Check sheet for the drawn part. Datum: minimum x, y, z corner. Units: mm. A direction names the side the tool comes from. Coordinates: 2 decimals unless noted, no trailing zeros. Write each loop counter-clockwise with the first axis right and the second up, starting at its lowest first coordinate (ties: lowest second). Pieces come first, ordered by that corner, then holes. Notation, with made-up numbers: (-20.75, 71.5) - (-1.75, 71.5) arc R21 cw to (-1.75, 79.5) - close; hole circle Ø11 at (-37.75, 39.25). An arc over 180 degrees is marked (long way). Use CSV: the item, a comma, the result in double quotes. Start each with the question number.
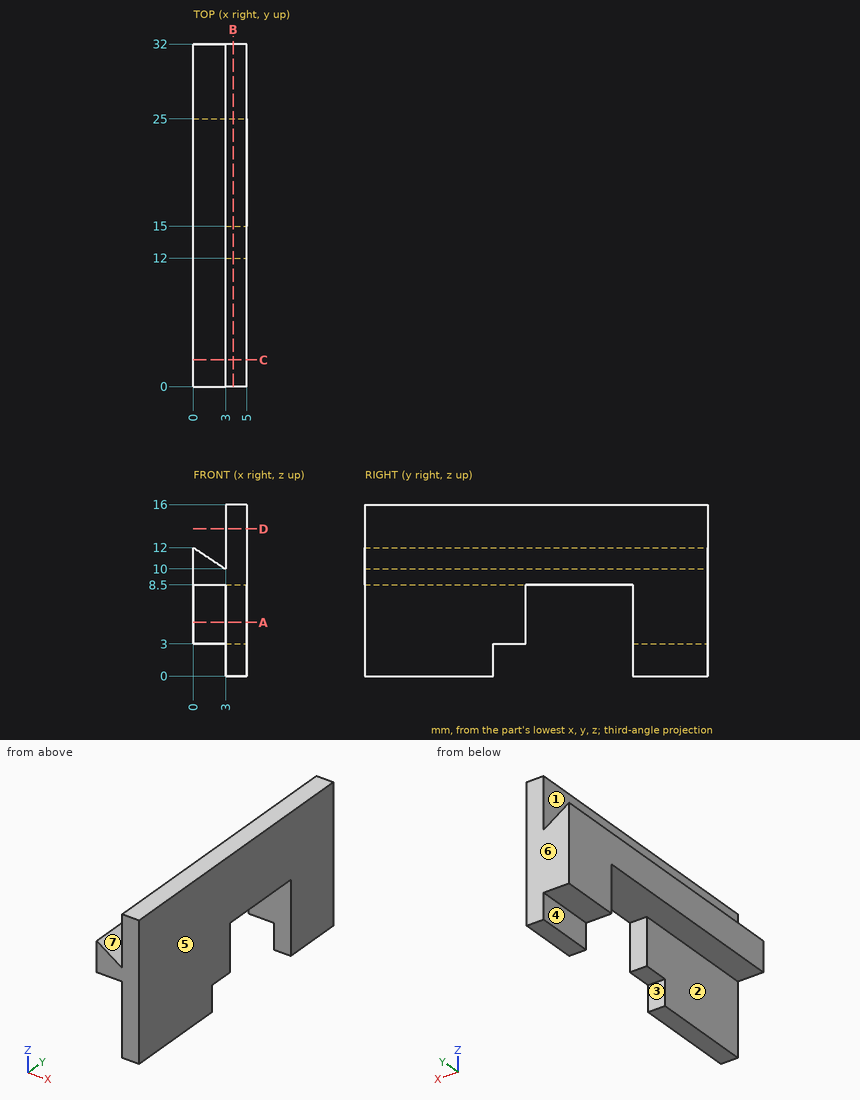
Q1. Cross-section at D-D (z = 13.75). Record the cut outline in (x, y), plus the area to 3 significant figures.
Q2. Cross-section at C-C (y = 2.5). Record the cut outline in (x, z), plus the area to 3 significant figures.
Q3. Tool access check on the marked faces 1, 2, 3 and 4. Record the directions out of +Z, -Z, +X, -X, +Y, -Y that give a thin tool (end or side, any length) a straight path to the whole face; none if there is none.
Q4. Cross-section at A-A (z = 5). Record the cut outline in (x, y).
Q5. Gauge pin test, flat ends, axial feed: pin 1 (2 mm diameter, centred on x = 4.5, y = 13.5, fed in from -Z); pin 2 (4 mm diameter, centred on y = 11, z = 5.5, fed in from -X). Record the tip position at first contact, or that the pin passes through.
Q6. Cross-section at B-B (x = 3.7). Record the cut outline in (y, z), plus the area to 3 significant figures.
Q7. Scan lines: line 1 along Y through (x, z) = (4.6, 2.5); line 2 along X through (y, z) = (20, 12.75); line 3 along Y through (x, z) = (4.6, 6.5). Record each from-to range of solid material in increasing order. Write a range as from..to.
Q8. Release check for a two-part mould opening along X. For the marked faces 5, 6 and 7 record: released by +X, released by -X, zero draft, split by the parting line, or undercut.
Reply:
1,outline,"(3, 0) - (5, 0) - (5, 32) - (3, 32) - close"
1,area,"64.0 mm^2"
2,outline,"(0, 8.5) - (3, 8.5) - (3, 0) - (5, 0) - (5, 16) - (3, 16) - (3, 10) - (0, 12) - close"
2,area,"39.5 mm^2"
3,face 1,"+Z, +Y, -Y"
3,face 2,"-Z, -X, -Y"
3,face 3,"-Z, +X, -X"
3,face 4,"-Z, -X, +Y, -Y"
4,outline,"(0, 25) - (5, 25) - (5, 32) - (0, 32) - close; (3, 0) - (5, 0) - (5, 15) - (3, 15) - close"
5,pin 1,"z = 3"
5,pin 2,"x = 3"
6,outline,"(0, 0) - (12, 0) - (12, 3) - (15, 3) - (15, 8.5) - (25, 8.5) - (25, 0) - (32, 0) - (32, 16) - (0, 16) - close"
6,area,"418 mm^2"
7,line 1,"0..12, 25..32"
7,line 2,"3..5"
7,line 3,"0..15, 25..32"
8,face 5,"released by +X"
8,face 6,"zero draft"
8,face 7,"undercut"
